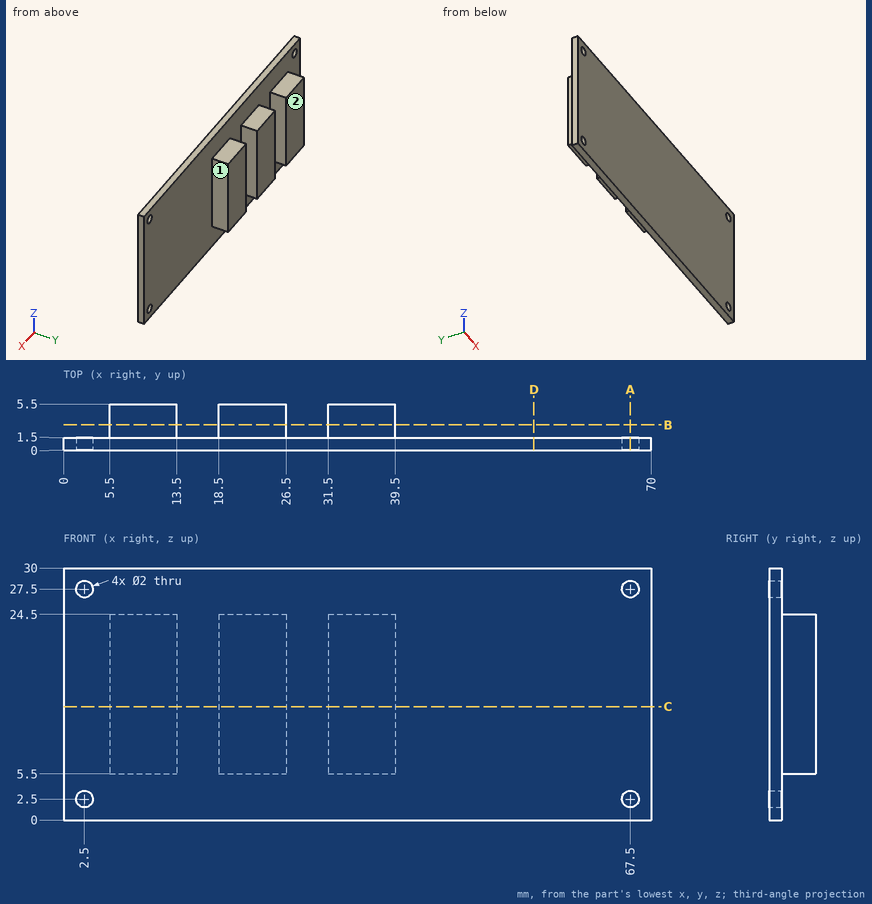
Answer from the drawing. Dimensions are ordinates in mm from the lowest x, y and z of the part. A direction names the side the tool comes from. Round coordinates to 2 decimals unless told otherwise and drop trailing zeros. Write each loop counter-clockwise with the first axis right and the second up, starting at its lowest first coordinate (ties: lowest second). Pieces come first, ordered by that corner, then holes. Notation, with made-up numbers: M 49,80 L 81,80 A12 cw 81,85 Z; hole C 28.5,-28.75 d9. An arc over 180 degrees is marked long. One line per item, written item: value.
Q1. Find section C-C on z = 13.5. Write down the section's boundary in (x, y).
Data:
outline: M 0,0 L 70,0 L 70,1.5 L 39.5,1.5 L 39.5,5.5 L 31.5,5.5 L 31.5,1.5 L 26.5,1.5 L 26.5,5.5 L 18.5,5.5 L 18.5,1.5 L 13.5,1.5 L 13.5,5.5 L 5.5,5.5 L 5.5,1.5 L 0,1.5 Z
Q2. Find section D-D on x = 56. Write down the section's boundary in (y, z).
Data:
outline: M 0,0 L 1.5,0 L 1.5,30 L 0,30 Z
Q3. Which of the six approach directions +Z, -Z, +X, -X, +Y, -Y give full straight-line access (tool end or side, diameter ignored) to the marked faces 1 and 2?
Data:
face 1: +Z, -Z, +X, +Y
face 2: +Z, -Z, +X, -X, +Y
Q4. Find section A-A on x = 67.5. Write down the section's boundary in (y, z), plus the area to 3 significant figures.
Data:
outline: M 0,0 L 1.5,0 L 1.5,1.5 L 0,1.5 Z; M 0,3.5 L 1.5,3.5 L 1.5,26.5 L 0,26.5 Z; M 0,28.5 L 1.5,28.5 L 1.5,30 L 0,30 Z
area: 39.0 mm2
Q5. Flat-ended cylindrical pins translate along their axes: pin 1 Ø2 at (x, y) = (36.5, 3.5) entering from -Z; pin 2 Ø1.2 at (x, z) = (2.5, 2.5) entering from -Y; pin 3 Ø2 at (x, y) = (12.5, 4.5) entering from +Z; pin 4 Ø3 at (y, z) = (4, 18) entering from +X. Find the tip coordinate at first contact, or state that the pin passes through.
Data:
pin 1: z = 5.5
pin 2: through
pin 3: z = 24.5
pin 4: x = 39.5
Q6. Find section B-B on y = 3. Write down the section's boundary in (x, z).
Data:
outline: M 5.5,5.5 L 13.5,5.5 L 13.5,24.5 L 5.5,24.5 Z; M 18.5,5.5 L 26.5,5.5 L 26.5,24.5 L 18.5,24.5 Z; M 31.5,5.5 L 39.5,5.5 L 39.5,24.5 L 31.5,24.5 Z
Q7. Straight lines are drawn through the part: line 1 (Z direction, x = 67.5, y = 1.05); line 2 (X direction, y = 5.05, z = 11.75); line 3 (X direction, y = 0.45, z = 27.5). For each, find the intervals that lie inside material, in ascending order. Write a range as [from, to].
Data:
line 1: [0, 1.5], [3.5, 26.5], [28.5, 30]
line 2: [5.5, 13.5], [18.5, 26.5], [31.5, 39.5]
line 3: [0, 1.5], [3.5, 66.5], [68.5, 70]
